Geometry: final body of the model. Coordinates: model frame, mm. Face numbers are marked on the shaded views. A direction names the side the tool comes from. Round coordinates to 2 decimals unless told otherwise and drop trailing zeros. Loops run counter-clockwise (first coordinate to the right, second up) from the corner with the lowest first, then second, coordinate; pieces in that order, holes last. Notation, with made-up numbers: M 14,78.25 L 59,78.25 A32 cw 59,114.25 Z; hole C 0.5,7.25 d6. An arc over 180 degrees is marked long. Answer as a JSON object with one key per item and string values.
```python
from build123d import *

# Parameters (mm, degrees)
BOSS_EXTRUDE1_DEPTH = 20
SKETCH2_W           = 13
SKETCH2_H           = 57
BOSS_EXTRUDE2_DEPTH = 30
SKETCH3_W           = 30
SKETCH3_H           = 20
CUT_EXTRUDE1_DEPTH  = 102.931349447
BOSS_EXTRUDE3_REACH = 118.931
BOSS_EXTRUDE3_START = -15
SKETCH5_W           = 20
SKETCH5_H           = 35


with BuildPart() as part:
    # Sketch1 → Boss-Extrude1 (new, symmetric)
    with BuildSketch(Plane.XY):
        Polygon((0, 0), (66, 0), (66, 57), (34, 57), (0, 15), align=None)
    extrude(amount=BOSS_EXTRUDE1_DEPTH, both=True)

    # Sketch2 → Boss-Extrude2 (add, symmetric)
    with BuildSketch(Plane.XY):
        with Locations((72.5, 28.5)):
            Rectangle(SKETCH2_W, SKETCH2_H)
    extrude(amount=BOSS_EXTRUDE2_DEPTH, both=True)

    # Sketch3 → Cut-Extrude1 (cut, through all)
    with BuildSketch(Plane(origin=(0, 0, 0), x_dir=(1, 0, 0), z_dir=(0, 1, 0))):
        with Locations((64, 0)):
            Rectangle(SKETCH3_W, SKETCH3_H)
    extrude(amount=CUT_EXTRUDE1_DEPTH, mode=Mode.SUBTRACT)

    # Sketch5 → Boss-Extrude3 (add, up to next)
    with BuildSketch(Plane(origin=(0, 0, 0), x_dir=(0, 0, -1), z_dir=(1, 0, 0)).offset(BOSS_EXTRUDE3_START), mode=Mode.PRIVATE) as boss_extrude3_sk1:
        with Locations((0, 17.5)):
            Rectangle(SKETCH5_W, SKETCH5_H)
    boss_extrude3_tool1 = extrude(boss_extrude3_sk1.sketch, amount=BOSS_EXTRUDE3_REACH, mode=Mode.PRIVATE) - part.part
    add(boss_extrude3_tool1.solids().sort_by_distance((-15, 17.5, 0))[0])


solid = part.part
```
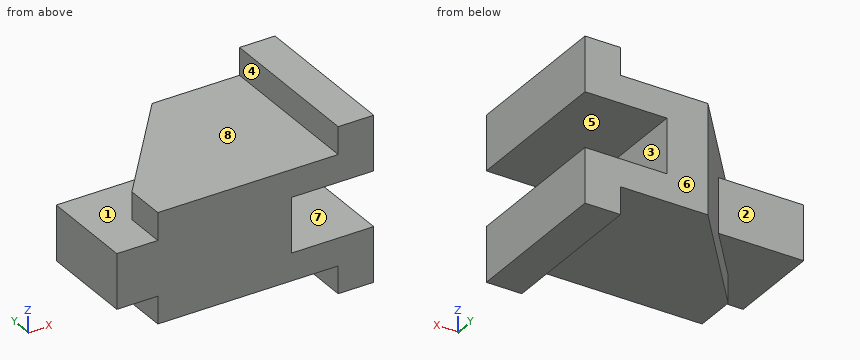
1) Cut plane C-C on z = 4. Return the cut outline in (x, y), and give its area (3 significant figures).
Geometry results:
{"outline": "M -15,0 L 49,0 L 49,57 L 34,57 L 16.19,35 L -15,35 Z", "area": "2,770 mm2"}
2) Cut plane D-D on x = 55.5. Return the cut outline in (y, z), and give its area (3 significant figures).
Geometry results:
{"outline": "M 0,-20 L 57,-20 L 57,-10 L 0,-10 Z; M 0,10 L 57,10 L 57,20 L 0,20 Z", "area": "1,140 mm2"}
3) Pull-direction query (Z, two-part tool) for the marked faces 5, 6, 7 and 8; classes: +Z half, -Z half, draft (parallel to the pull), parting line (faces both ways), or undercut.
Geometry results:
{"face 5": "undercut", "face 6": "draft", "face 7": "undercut", "face 8": "+Z half"}
4) Cut plane B-B on y = 25.5. Return the cut outline in (x, z).
Geometry results:
{"outline": "M -15,-10 L 8.5,-10 L 8.5,-20 L 66,-20 L 66,-30 L 79,-30 L 79,-10 L 49,-10 L 49,10 L 79,10 L 79,30 L 66,30 L 66,20 L 8.5,20 L 8.5,10 L -15,10 Z"}
5) Cut plane A-A on x = 73.5. Return the cut outline in (y, z), and give its area (3 significant figures).
Geometry results:
{"outline": "M 0,-30 L 57,-30 L 57,-10 L 0,-10 Z; M 0,10 L 57,10 L 57,30 L 0,30 Z", "area": "2,280 mm2"}
6) Line query: probe 1 along Z at (x, y) = (71.5, 25.5); probe 2 along Z at (x, y) = (59, 39.5); probe 3 along X at (y, z) = (26, 0). Output: solid intervals per line, ascending.
Geometry results:
{"probe 1": "-30 to -10, 10 to 30", "probe 2": "-20 to -10, 10 to 20", "probe 3": "-15 to 49"}
7) Set-up query: the marked faces 1, 2, 3 and 4. Return all of +Z, -Z, +X, -X, +Y, -Y with unobstructed straight access to the full face (end or side cutting, diameter ignored); none if empty.
Geometry results:
{"face 1": "+Z, -X, +Y", "face 2": "+Z, -Z, -X, +Y", "face 3": "+X, +Y, -Y", "face 4": "+Z, -X, +Y, -Y"}
8) First-contact query: pin 1 (10 mm diameter, centred on y = 15, z = -0.5, fed in from +X); pin 2 (9.5 mm diameter, centred on x = 6.5, y = 14.5, fed in from -Z); pin 3 (10 mm diameter, centred on x = 0, z = -10, fed in from +Y); pin 4 (5 mm diameter, centred on x = 3.5, z = 20, fed in from -Y). Flat tips, straight axial feed; report the tip coordinate or a pass-through.
Geometry results:
{"pin 1": "x = 49", "pin 2": "z = -20", "pin 3": "y = 35", "pin 4": "y = 0"}
